Can you work these out from the model? Positions are in its coordinate system, mm. A direction names the side the tool comes from. Give positions to 0.01 mm unless a question says otherwise; leave off trailing zeros. Order: outer loops, then holes, each group sorted by start corner. A loop starts at its lowest first (then second) coordinate and runs counter-clockwise, first axis right, second up. Notation, with made-up numbers: M 67.5,69 L 77.5,69 A18 ccw 77.5,80 Z; hole C 29,8 d6. An arc over 180 degrees is marked long. Write each question's results on one line, items separated by ' | '.
from build123d import *

# Parameters (mm, degrees)
SKETCH_1_R      = 5.25
SKETCH_1_R_2    = 1.5
SKETCH_1_R_3    = 3
EXTRUDE_1_DEPTH = 3
FILLET_1_R      = 10
FILLET_2_R      = 15


with BuildPart() as part:
    # 草图1 → 凸台-拉伸1 (new body)
    with BuildSketch(Plane.XY):
        Polygon((94.821200219, 20), (69.821200219, 20), (40, 30), (0, 30), (0, 0), (94.821200219, 0), align=None)
        with Locations((15, 15)):
            Circle(SKETCH_1_R, mode=Mode.SUBTRACT)
        with Locations((15, 23)):
            Circle(SKETCH_1_R_2, mode=Mode.SUBTRACT)
        with Locations((15, 7)):
            Circle(SKETCH_1_R_2, mode=Mode.SUBTRACT)
        with Locations((23, 15)):
            Circle(SKETCH_1_R_2, mode=Mode.SUBTRACT)
        with Locations((7, 15)):
            Circle(SKETCH_1_R_2, mode=Mode.SUBTRACT)
        with Locations((84.821200219, 10)):
            Circle(SKETCH_1_R_3, mode=Mode.SUBTRACT)
    extrude(amount=EXTRUDE_1_DEPTH)

    # 圆角1
    fillet_1_edges = [part.edges().sort_by_distance(p)[0] for p in [
        (94.821200219, 0, 1.5),
        (94.821200219, 20, 1.5),
        (69.821200219, 20, 1.5),
        (40, 30, 1.5),
    ]]
    fillet(fillet_1_edges, radius=FILLET_1_R - 0.0001)  # a hair under: the kernel refuses the full size

    # 圆角2
    fillet_2_edges = [part.edges().sort_by_distance(p)[0] for p in [
        (0, 0, 1.5),
        (0, 30, 1.5),
    ]]
    fillet(fillet_2_edges, radius=FILLET_2_R - 0.0001)  # a hair under: the kernel refuses the full size


solid = part.part
(1) Imagine slicing it at C-C, the plane y = 23. Write out the boundary of the cut face in (x, z), plus the area to 3 significant figures.
Data:
outline: M 2.31,0 L 13.5,0 L 13.5,3 L 2.31,3 Z; M 16.5,0 L 60.87,0 L 60.87,3 L 16.5,3 Z | area: 167 mm2
(2) I need wall thicknesses on L1, parallel to Y at x = 15, z = 1.95; L2, parallel to Y at x = 23, z = 1.25; L3, parallel to X at y = 12, z = 2.75. Which ranges of each line are inside material? Lowest first, please. Write a range as from..to.
Data:
L1: y = 0..5.5, 8.5..9.75, 20.25..21.5, 24.5..30 | L2: y = 0..13.5, 16.5..30 | L3: x = 0.3..10.69, 19.31..82.59, 87.06..94.62
(3) Imagine slicing it at B-B, the plane z = 2.05. Count the separate pieces of the cut face and the enclosed holes in it, plus the area to 3 significant figures.
Data:
separate pieces: 1 | enclosed holes: 6 | area: 2,160 mm2
(4) We'd pull the mould along Y, two halves only. Please class faces 3 (the face through (91.97, 3.01, 1.52)), 4 (the face through (40.001, 29.866, 1.521)), 5 (the face through (13.89, 24.01, 1.48)), 6 (the face through (21.5, 15.07, 1.48)): +Y half, -Y half, draft (parallel to the pull), parting line (faces both ways), or undercut.
Data:
face 3: -Y half | face 4: +Y half | face 5: undercut | face 6: undercut
(5) For faces 1 (the face through (78, 20, 1)), 2 (the face through (47, 12, 0)), which set-ups out of +Z, -Z, +X, -X, +Y, -Y let a thin tool reach every point of the face, with its end or its side?
Data:
face 1: +Z, -Z, +X, +Y | face 2: -Z, +X, -X, +Y, -Y
(6) Will this pin go through, and if not, where does the flat tip stop? P1, Ø1.5, axis at x = 79, z = 2, coming from the +Y side.
Data:
P1: stops at y = 20
(7) Imagine slicing it at A-A, the plane x = 23. Write out the boundary of the cut face in (y, z), plus the area to 3 significant figures.
Data:
outline: M 0,0 L 13.5,0 L 13.5,3 L 0,3 Z; M 16.5,0 L 30,0 L 30,3 L 16.5,3 Z | area: 81.0 mm2
(8) Imagine slicing it at D-D, the plane y = 11. Write out the boundary of the cut face in (x, z), plus the area to 3 significant figures.
Data:
outline: M 0.54,0 L 11.6,0 L 11.6,3 L 0.54,3 Z; M 18.4,0 L 81.99,0 L 81.99,3 L 18.4,3 Z; M 87.65,0 L 94.77,0 L 94.77,3 L 87.65,3 Z | area: 245 mm2
